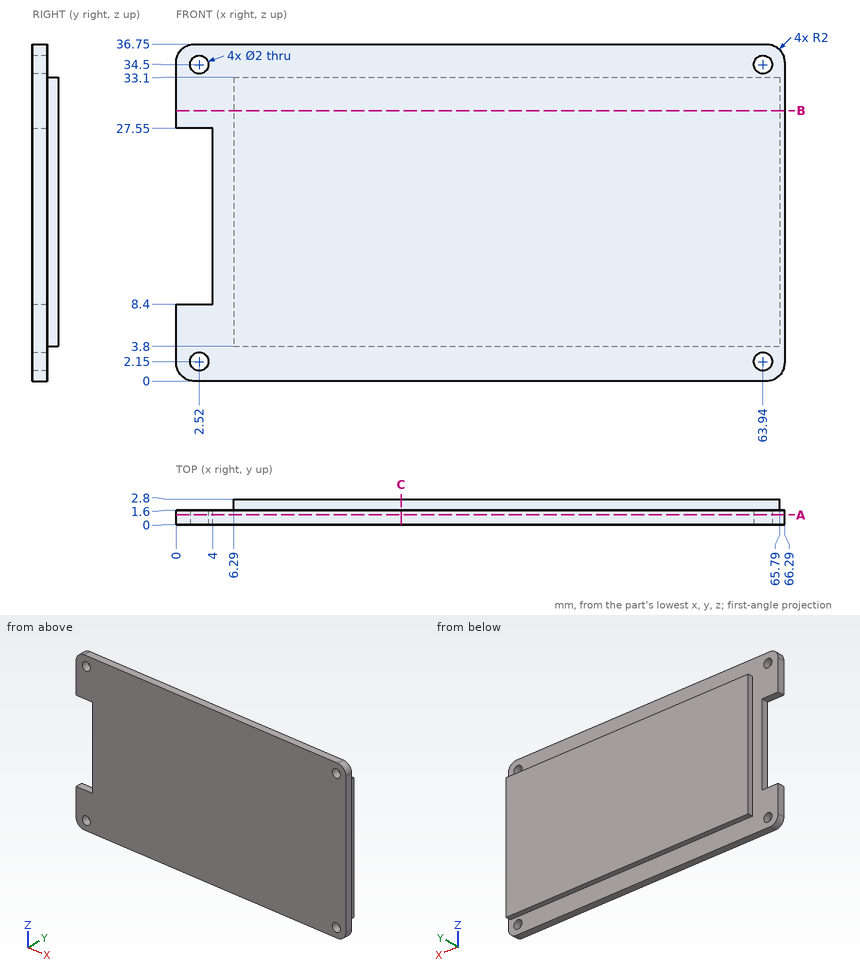
Design review of the part shown in the three views and the two pictorial views. Dimensions are in mm from the part's minimum x, y and z. Coordinates: 2 decimals unless noted, no trailing zeros. Order: outer loops, then holes, each group sorted by start corner. A loop starts at its lowest first (then second) coordinate and runs counter-clockwise, first axis right, second up.
Item 1: Take a section at A-A, the plane y = 1.1. Write out the cut boundary in (x, z).
Item 2: Take a section at C-C, the plane x = 24.5. Write out the cut boundary in (y, z).
Item 3: Take a section at B-B, the plane z = 29.5. Write out the cut boundary in (x, y).
Item 4: For pin 1 Ø1.3 at (y, z) = (2, 14) entering from -X; pin 2 Ø2.5 at (x, z) = (2.52, 2.15) entering from +Y, all flat-tipped, find the tip position at first contact; note any pin that passes through.
Item 5: For line 1 (X direction, y = 1.25, z = 34.5); line 2 (X direction, y = 0.4, z = 13); line 3 (Y direction, x = 52.5, z = 3), list the stretches that pass through material, from the lowest coordinate up.
The answers:
1. outline: (0, 2) arc R2 ccw to (2, 0) - (64.29, 0) arc R2 ccw to (66.29, 2) - (66.29, 34.75) arc R2 ccw to (64.29, 36.75) - (2, 36.75) arc R2 ccw to (0, 34.75) - (0, 27.55) - (4, 27.55) - (4, 8.4) - (0, 8.4) - close; hole circle Ø2 at (2.52, 2.15); hole circle Ø2 at (2.52, 34.5); hole circle Ø2 at (63.94, 2.15); hole circle Ø2 at (63.94, 34.5)
2. outline: (0, 0) - (1.6, 0) - (1.6, 3.8) - (2.8, 3.8) - (2.8, 33.1) - (1.6, 33.1) - (1.6, 36.75) - (0, 36.75) - close
3. outline: (0, 0) - (66.29, 0) - (66.29, 1.6) - (65.79, 1.6) - (65.79, 2.8) - (6.29, 2.8) - (6.29, 1.6) - (0, 1.6) - close
4. pin 1: stops at x = 4
4. pin 2: stops at y = 1.6
5. line 1: x = 0 to 1.52, 3.52 to 62.94, 64.94 to 66.29
5. line 2: x = 4 to 66.29
5. line 3: y = 0 to 1.6
